Source: CAD feature listing. Evaluate the final solid. Frame: model axes, mm. Round coordinates to 2 decimals unless told otherwise and drop trailing zeros. Loops run counter-clockwise (first coordinate to the right, second up) from the corner with the lowest first, then second, coordinate; pieces in that order, holes last.
(1) Section A-A, the plane y = 3. Return the cut outline in (x, z).
(2) Section B-B, the plane x = 14. Return the cut outline in (y, z).
(3) Section D-D, the plane x = 52. Return the cut outline in (y, z).
(4) Mould query, pull axis X, two halves, no side actions, for faces 1 (the cylindrical face through (-27, 1, 30)), 2 (the flat face through (13, -6, 0)), 3 (the flat face through (-36, 0, 30)). Classes: pulls with the +X half, pulls with the -X half, needs draft (parallel to the pull), parting line crosses it, or undercut.
(5) Section C-C, the plane z = 12. Return the cut outline in (x, y).
(6) First-contact query: pin 1 Ø1.5 at (x, y) = (-6, -20.5) entering from -Z. Flat tip, straight axial feed; report the tip coordinate or a pass-through.
(7) Material intervals for probe 1 along X at (y, z) = (-10, 30); probe 2 along Z at (x, y) = (-24, 7); probe 3 along Y at (x, z) = (16.5, 14), sorted ascending.
Autodesk Inventor part; units mm, degrees
ref_plane "YZ Plane" through (0, 0, 0) normal (1, 0, 0) x (0, 1, 0)
ref_plane "XZ Plane" through (0, 0, 0) normal (0, 1, 0) x (-1, 0, 0)
ref_plane "XY Plane" through (0, 0, 0) normal (0, 0, 1) x (1, 0, 0)
sketch "Sketch1" plane through (0, 0, 0) normal (0, 0, 1) x (1, 0, 0)
  line L0 (-36, 33) -> (64, 33)
  line L1 (64, 33) -> (64, -32)
  line L2 (64, -32) -> (-36, -32)
  line L3 (-36, -32) -> (-36, 33)
  point P0 (0, 0)
  dimension "d0" = 100
  dimension "d1" = 65
extrude "Extrusion1" add sketch "Sketch1" along normal blind 60
sketch "Sketch2" plane through (0, 0, 60) normal (0, 0, 1) x (1, 0, 0)
  circle A0 centre (14, 3) radius 8
  line L0 (64, 33) -> (-36, 33)
  line L1 (64, -32) -> (64, 33)
  line L2 (-36, -32) -> (64, -32)
  point P0 (0, 0)
  dimension "d4" = 16
  dimension "d6" = 50
  dimension "d7" = 35
extrude "Extrusion2" cut sketch "Sketch2" against normal through all
sketch "Sketch3" plane through (-36, 33, 0) normal (0, 1, 0) x (1, 0, 0)
  circle A0 centre (12, -30) radius 3
  line L0 (100, 0) -> (0, 0)
  line L1 (0, 0) -> (0, -60)
  circle A1 centre (88, -30) radius 3
  line L2 (100, 0) -> (100, -60)
  point P0 (36, 0)
  dimension "d10" = 6
  dimension "d11" = 30
  dimension "d12" = 12
  dimension "d13" = 6
  dimension "d14" = 30
  dimension "d15" = 12
extrude "Extrusion3" cut sketch "Sketch3" against normal through all
properties part number "Pin Block" material "Brass, Soft Yellow, Welded"
Output values:
1. outline: (-36, 0) - (6, 0) - (6, 60) - (-36, 60) - close; (22, 0) - (64, 0) - (64, 60) - (22, 60) - close; hole circle Ø6 at (-24, 30); hole circle Ø6 at (52, 30)
2. outline: (-32, 0) - (-5, 0) - (-5, 60) - (-32, 60) - close; (11, 0) - (33, 0) - (33, 60) - (11, 60) - close
3. outline: (-32, 0) - (33, 0) - (33, 27) - (-32, 27) - close; (-32, 33) - (33, 33) - (33, 60) - (-32, 60) - close
4. face 1: undercut
4. face 2: needs draft
4. face 3: pulls with the -X half
5. outline: (-36, -32) - (64, -32) - (64, 33) - (-36, 33) - close; hole circle Ø16 at (14, 3)
6. pin 1: stops at z = 0
7. probe 1: x = -36 to -27, -21 to 49, 55 to 64
7. probe 2: z = 0 to 27, 33 to 60
7. probe 3: y = -32 to -4.6, 10.6 to 33
